Print and shaded views of the part. All mm, measured from the part's lowest x, y and z. A direction names the side the tool comes from. Round coordinates to 2 decimals unless told otherwise and drop trailing zeros. Order: outer loops, then holes, each group sorted by start corner. A loop starts at its lowest first (then second) coordinate and runs counter-clockwise, first axis right, second up. Notation, with made-up numbers: M -6.75,-4 L 42.25,-4 A30 ccw 42.25,21 Z; hole C 54.25,-19.75 d3. An arc over 180 degrees is marked long. Use CSV: the item, a comma, the result in double quotes.
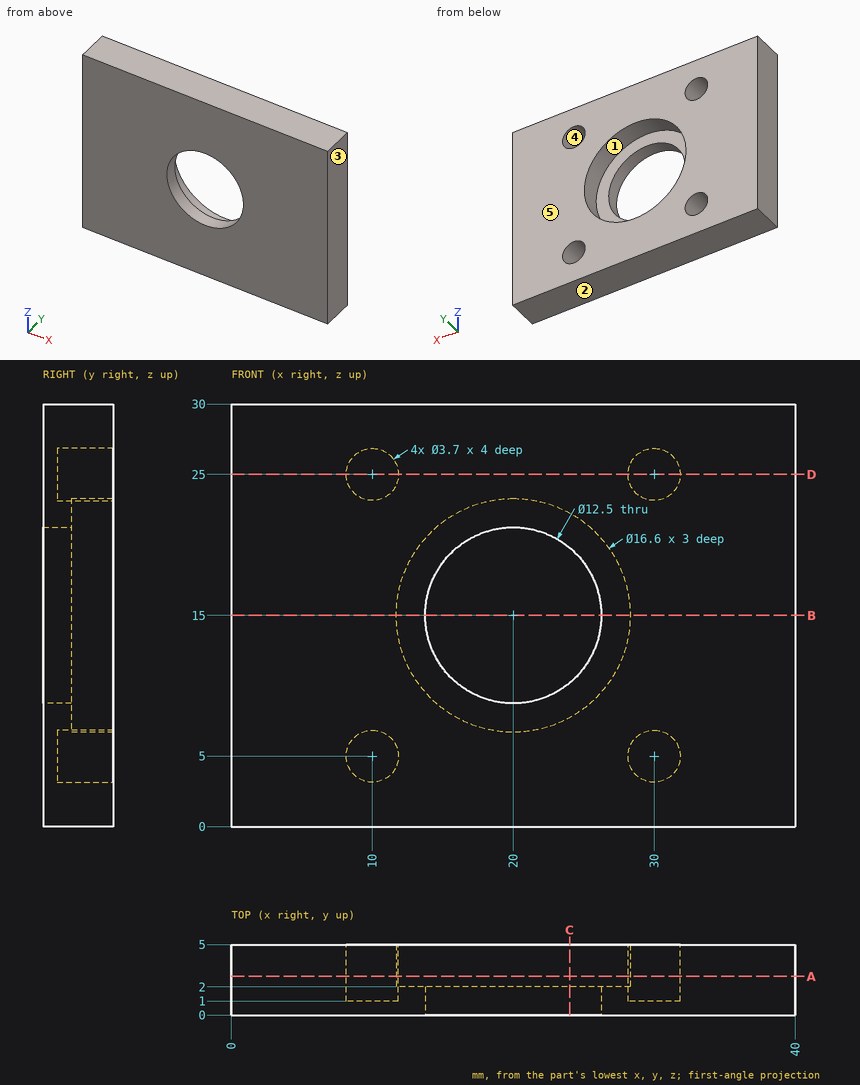
(1) Cut at C-C, the plane x = 24. Give the cut face in (y, z).
Answer block:
outline,"M 0,0 L 5,0 L 5,7.73 L 2,7.73 L 2,10.2 L 0,10.2 Z; M 0,19.8 L 2,19.8 L 2,22.27 L 5,22.27 L 5,30 L 0,30 Z"
(2) Cut at B-B, the plane z = 15. Give the cut face in (x, y).
Answer block:
outline,"M 0,0 L 13.75,0 L 13.75,2 L 11.7,2 L 11.7,5 L 0,5 Z; M 26.25,0 L 40,0 L 40,5 L 28.3,5 L 28.3,2 L 26.25,2 Z"
(3) Cut at D-D, the plane z = 25. Give the cut face in (x, y).
Answer block:
outline,"M 0,0 L 40,0 L 40,5 L 31.85,5 L 31.85,1 L 28.15,1 L 28.15,5 L 11.85,5 L 11.85,1 L 8.15,1 L 8.15,5 L 0,5 Z"
(4) Tool access for the marked faces 1 and 2: list every direction of +Z, -Z, +X, -X, +Y, -Y with a clear straight run to the whole face (end or side of a thin tool).
Answer block:
face 1,"+Y"
face 2,"-Z, +X, -X, +Y, -Y"
(5) Two-plate mould, pull along X, no slides. Class the marked faces 3, 4 and 5: released by +X, released by -X, zero draft, split by the parting line, or undercut.
Answer block:
face 3,"released by +X"
face 4,"undercut"
face 5,"zero draft"
(6) Drop a flat-ended pin along its axis: pin 1 (2 mm diameter, centred on x = 30, z = 5, fed in from +Y). Give the stop position or say it passes through.
Answer block:
pin 1,"stops at y = 1"
(7) Wall check: line 1 (X direction, y = 3.55, z = 5); line 2 (X direction, y = 1.4, z = 4); line 3 (X direction, y = 1.6, z = 15). Give the ranges that are in metal, low to high. Write a range as from..to.
Answer block:
line 1,"x = 0..8.15, 11.85..28.15, 31.85..40"
line 2,"x = 0..8.44, 11.56..28.44, 31.56..40"
line 3,"x = 0..13.75, 26.25..40"
(8) Cut at A-A, the plane y = 2.75. Give the cut face in (x, z), and give its area (3 significant figures).
Answer block:
outline,"M 0,0 L 40,0 L 40,30 L 0,30 Z; hole C 10,5 d3.7; hole C 10,25 d3.7; hole C 20,15 d16.6; hole C 30,5 d3.7; hole C 30,25 d3.7"
area,"941 mm²"
